Geometry: final body of the model. Coordinates: model frame, mm. A direction names the side the tool comes from. Give positions to 0.01 mm unless a question says otherwise; leave off trailing zeros. Write each loop counter-clockwise with the first axis right and the second up, starting at its lowest first coordinate (ties: lowest second). Pieces come first, ordered by that corner, then holes.
Q1. Section C-C (z = 16.5). Return the cut outline in (x, y), plus the area to 3 significant figures.
Q2. Section D-D (y = -22). Return the cut outline in (x, z), plus the area to 3 significant figures.
Q3. Line query: line 1 (Y direction, x = 17.5, z = 21.4); line 2 (Y direction, x = 17.5, z = 22.5); line 3 (Y direction, x = 17.5, z = 6.5). Output: solid intervals per line, ascending.
Q4. Reachability of faces 1 (the flat face through (0, -18, 11)), 2 (the cylindrical face through (29.66, -21.33, 9.37)), 3 (the cylindrical face through (15.29, -6.47, 22.41)) from +Z, -Z, +X, -X, +Y, -Y: full face, straight path, thin tool, end or side. Return the list, or none.
Q5. Mould query, pull axis Y, two halves, no side actions, for faces 4 (the flat face through (6, -9, 0)), 5 (the flat face through (16, -28, 21.8)), 6 (the flat face through (17, 0, 11)). Classes: +Y half, -Y half, draft (parallel to the pull), parting line (faces both ways), or undercut.
Q6. Section A-A (y = -17.5). Return the cut outline in (x, z), plus the area to 4 significant figures.
Q7. Pin query (flat end, axial travel): pin 1 Ø2 at (x, y) = (17.5, -8.5) entering from -Z; pin 2 Ø1.8 at (x, y) = (18, -25) entering from +Z; pin 3 Ø15.5 at (x, y) = (17.5, -17.5) entering from -Z. Return the tip coordinate at first contact, or that it passes through.
Q8. Section B-B (x = 17.5). Return the cut outline in (y, z), plus the area to 3 significant figures.
Autodesk Inventor part; units mm, degrees
ref_plane "YZ Plane" through (0, 0, 0) normal (1, 0, 0) x (0, 1, 0)
ref_plane "XZ Plane" through (0, 0, 0) normal (0, 1, 0) x (-1, 0, 0)
ref_plane "XY Plane" through (0, 0, 0) normal (0, 0, 1) x (1, 0, 0)
sketch "Sketch1" plane through (0, 0, 0) normal (0, 0, 1) x (1, 0, 0)
  line L0 (0, 0) -> (35, 0)
  line L1 (35, 0) -> (35, -35)
  line L2 (35, -35) -> (0, -35)
  line L3 (0, -35) -> (0, 0)
  circle A0 centre (17.5, -17.5) radius 12.75
  dimension "d0" = 35
  dimension "d1" = 35
  dimension "d2" = 25.5
extrude "Extrusion1" add sketch "Sketch1" along normal blind 19
sketch "Sketch2" plane through (0, 0, 19) normal (0, 0, 1) x (1, 0, 0)
  line L0 (35, -35) -> (35, 0)
  line L1 (0, 0) -> (35, 0)
  line L2 (35, 0) -> (35, -35)
  line L3 (35, -35) -> (0, -35)
  line L4 (0, -35) -> (0, 0)
  circle A0 centre (17.5, -17.5) radius 3.75
  circle A1 centre (17.5, -8.5) radius 1.85
  circle A2 centre (17.5, -26.5) radius 1.85
  dimension "d5" = 7.5
  dimension "d6" = 17.5
  dimension "d7" = 17.5
  dimension "d8" = 3.7
  dimension "d9" = 3.7
  dimension "d10" = 9
  dimension "d11" = 9
extrude "Extrusion2" add sketch "Sketch2" along normal blind 4
sketch "Sketch3" plane through (0, 0, 23) normal (0, 0, 1) x (1, 0, 0)
  circle A0 centre (17.5, -8.5) radius 1.85
  circle A1 centre (17.5, -8.5) radius 3
  circle A2 centre (17.5, -26.5) radius 1.85
  circle A3 centre (17.5, -26.5) radius 3
  point P0 (0, 0)
  dimension "d14" = 6
  dimension "d15" = 6
extrude "Extrusion3" cut sketch "Sketch3" against normal blind 1.2
properties part number "Motor_Support"
Computed:
1. outline: (0, -35) - (35, -35) - (35, 0) - (0, 0) - close; hole circle Ø25.5 at (17.5, -17.5)
1. area: 714 mm2
2. outline: (0, 0) - (5.57, 0) - (5.57, 19) - (29.43, 19) - (29.43, 0) - (35, 0) - (35, 23) - (0, 23) - close
2. area: 352 mm2
3. line 1: y = -35 to -28.35, -24.65 to -21.25, -13.75 to -10.35, -6.65 to 0
3. line 2: y = -35 to -29.5, -23.5 to -21.25, -13.75 to -11.5, -5.5 to 0
3. line 3: y = -35 to -30.25, -4.75 to 0
4. face 1: +Z, -Z, -X, +Y, -Y
4. face 2: -Z
4. face 3: +Z
5. face 4: draft
5. face 5: undercut
5. face 6: +Y half
6. outline: (0, 0) - (4.75, 0) - (4.75, 19) - (13.75, 19) - (13.75, 23) - (0, 23) - close; (21.25, 19) - (30.25, 19) - (30.25, 0) - (35, 0) - (35, 23) - (21.25, 23) - close
6. area: 290.5 mm2
7. pin 1: passes through
7. pin 2: stops at z = 21.8
7. pin 3: stops at z = 19
8. outline: (-35, 0) - (-30.25, 0) - (-30.25, 19) - (-28.35, 19) - (-28.35, 21.8) - (-29.5, 21.8) - (-29.5, 23) - (-35, 23) - close; (-24.65, 19) - (-21.25, 19) - (-21.25, 23) - (-23.5, 23) - (-23.5, 21.8) - (-24.65, 21.8) - close; (-13.75, 19) - (-10.35, 19) - (-10.35, 21.8) - (-11.5, 21.8) - (-11.5, 23) - (-13.75, 23) - close; (-6.65, 19) - (-4.75, 19) - (-4.75, 0) - (0, 0) - (0, 23) - (-5.5, 23) - (-5.5, 21.8) - (-6.65, 21.8) - close
8. area: 255 mm2
